Design review of the part built by this model. Coordinates are the model's own, in mm. A direction names the side the tool comes from. Give positions to 0.01 mm unless a question says otherwise; leave off trailing zeros. Order: outer loops, then holes, each group sorted by start corner. A loop starts at its lowest first (then second) coordinate and runs counter-clockwise, first axis right, second up. Notation, with made-up numbers: (83.25, -10) -> (139.25, -10) arc R30 cw to (139.25, 14) -> close; hole circle Ø7 at (29.25, 7.5). An arc over 180 degrees is marked (long way). Return JSON: item names as keys, results as strings.
```python
from build123d import *

# Parameters (mm, degrees)
SKETCH_1_W          = 16.3
SKETCH_1_H          = 31.2
SKETCH_1_R          = 3.05
SKETCH_1_R_2        = 1.05
SKETCH_1_R_3        = 2.55
EXTRUDE_1_DEPTH     = 2.5
SKETCH_2_R          = 1
CUT_EXTRUDE_1_DEPTH = 1
SKETCH_2_3_R        = 0.7
CUT_EXTRUDE_2_DEPTH = 21.5655051
SKETCH_3_R          = 1.5
SKETCH_3_R_2        = 2.5
EXTRUDE_2_DEPTH     = 9
CUT_EXTRUDE_START   = 9
SKETCH_3_3_R        = 0.3
CUT_EXTRUDE_3_DEPTH = 2
SKETCH_4_R          = 0.3
CUT_EXTRUDE_4_DEPTH = 2


with BuildPart() as part:
    # 草图1 → 凸台-拉伸1 (new body)
    with BuildSketch(Plane(origin=(0, 0, 0), x_dir=(1, 0, 0), z_dir=(0, 1, 0))):
        with Locations((3.15, 1.4)):
            Rectangle(SKETCH_1_W, SKETCH_1_H)
        with Locations(Location((0, 0, 0), (0, 0, 270))):
            Circle(SKETCH_1_R, mode=Mode.SUBTRACT)
        with Locations(Location((5.25646039, -8.152277238, 0), (0, 0, 270))):
            Circle(SKETCH_1_R_2, mode=Mode.SUBTRACT)
        with Locations(Location((6.4, -3.8, 0), (0, 0, 270))):
            Circle(SKETCH_1_R, mode=Mode.SUBTRACT)
        with Locations(Location((-0.337099263, 6.891760594, 0), (0, 0, 270))):
            Circle(SKETCH_1_R_3, mode=Mode.SUBTRACT)
        with Locations(Location((4.7, 11, 0), (0, 0, 270))):
            Circle(SKETCH_1_R_3, mode=Mode.SUBTRACT)
    extrude(amount=EXTRUDE_1_DEPTH)

    # 草图2 → 切除-拉伸1 (cut)
    with BuildSketch(Plane(origin=(0, 2.5, 0), x_dir=(1, 0, 0), z_dir=(0, 1, 0))):
        with Locations(Location((-3.5, 15.5, 0), (0, 0, 270))):
            Circle(SKETCH_2_R)
        with Locations(Location((-3.5, -12.7, 0), (0, 0, 270))):
            Circle(SKETCH_2_R)
        with Locations(Location((9.8, -12.7, 0), (0, 0, 270))):
            Circle(SKETCH_2_R)
        with Locations(Location((9.8, 15.5, 0), (0, 0, 270))):
            Circle(SKETCH_2_R)
        with Locations(Location((-3.5, -6.5, 0), (0, 0, 270))):
            Circle(SKETCH_2_R)
        with Locations(Location((9.8, 0, 0), (0, 0, 270))):
            Circle(SKETCH_2_R)
        with Locations(Location((9.8, 6.5, 0), (0, 0, 270))):
            Circle(SKETCH_2_R)
    extrude(amount=-CUT_EXTRUDE_1_DEPTH, mode=Mode.SUBTRACT)

    # 草图2<3> → 切除-拉伸2 (cut, through all)
    with BuildSketch(Plane(origin=(0, 2.5, 0), x_dir=(1, 0, 0), z_dir=(0, 1, 0))):
        with Locations(Location((9.8, 15.5, 0), (0, 0, 270))):
            Circle(SKETCH_2_3_R)
        with Locations(Location((9.8, -12.7, 0), (0, 0, 270))):
            Circle(SKETCH_2_3_R)
        with Locations(Location((-3.5, -12.7, 0), (0, 0, 270))):
            Circle(SKETCH_2_3_R)
        with Locations(Location((-3.5, 15.5, 0), (0, 0, 270))):
            Circle(SKETCH_2_3_R)
        with Locations(Location((-3.5, -6.5, 0), (0, 0, 270))):
            Circle(SKETCH_2_3_R)
        with Locations(Location((9.8, 0, 0), (0, 0, 270))):
            Circle(SKETCH_2_3_R)
        with Locations(Location((9.8, 6.5, 0), (0, 0, 270))):
            Circle(SKETCH_2_3_R)
    extrude(amount=-CUT_EXTRUDE_2_DEPTH, mode=Mode.SUBTRACT)

    # 草图3 → 凸台-拉伸2 (add)
    with BuildSketch(Plane(origin=(0, 2.5, 0), x_dir=(1, 0, 0), z_dir=(0, 1, 0))):
        with Locations(Location((-3.5, -9.6, 0), (0, 0, 180))):
            Circle(SKETCH_3_R)
        with Locations(Location((-3.5, 12, 0), (0, 0, 180))):
            Circle(SKETCH_3_R)
        with Locations(Location((6.3, 4, 0), (0, 0, 90))):
            Circle(SKETCH_3_R_2)
        with Locations((9.8, 11)):
            Circle(SKETCH_3_R)
    extrude(amount=EXTRUDE_2_DEPTH)

    # 草图3<3> → 切除-拉伸3 (cut)
    with BuildSketch(Plane(origin=(0, 2.5, 0), x_dir=(1, 0, 0), z_dir=(0, 1, 0)).offset(CUT_EXTRUDE_START)):
        with Locations(Location((-3.5, -9.6, 0), (0, 0, 270))):
            Circle(SKETCH_3_3_R)
        with Locations(Location((-3.5, 12, 0), (0, 0, 270))):
            Circle(SKETCH_3_3_R)
        with Locations(Location((6.3, 4, 0), (0, 0, 270))):
            Circle(SKETCH_3_3_R)
        with Locations(Location((9.8, 11, 0), (0, 0, 270))):
            Circle(SKETCH_3_3_R)
    extrude(amount=-CUT_EXTRUDE_3_DEPTH, mode=Mode.SUBTRACT)

    # 草图4 → 切除-拉伸4 (cut)
    with BuildSketch(Plane(origin=(0, 0, -17), x_dir=(-1, 0, 0), z_dir=(0, 0, -1))):
        with Locations((0.8, 1.187263162)):
            Circle(SKETCH_4_R)
        with Locations((-4.2, 1.187263162)):
            Circle(SKETCH_4_R)
    extrude(amount=-CUT_EXTRUDE_4_DEPTH, mode=Mode.SUBTRACT)


solid = part.part
```
Item 1: Add section B-B (z = 0). Give the boundary of the cut face in (x, y).
Result set:
{"outline": "(-5, 0) -> (-3.05, 0) -> (-3.05, 2.5) -> (-5, 2.5) -> close; (3.05, 0) -> (9.1, 0) -> (9.1, 1.5) -> (8.8, 1.5) -> (8.8, 2.5) -> (3.05, 2.5) -> close; (10.5, 0) -> (11.3, 0) -> (11.3, 2.5) -> (10.8, 2.5) -> (10.8, 1.5) -> (10.5, 1.5) -> close"}
Item 2: Machinability: for faces 4 (the face through (-3.2, 2.007, -14.546)), 5 (the face through (-4, 11.5, 10)), which of the approach directions +Z, -Z, +X, -X, +Y, -Y give a long, thin tool a straight path to every point of the face, cutting with its end or side? Answer none if there is none.
Result set:
{"face 4": "+Y", "face 5": "+Z, -Z, +X, -X, +Y"}
Item 3: Add section D-D (x = 0). Give the boundary of the cut face in (y, z).
Result set:
{"outline": "(0, -17) -> (2.5, -17) -> (2.5, -9.42) -> (0, -9.42) -> close; (0, -4.36) -> (2.5, -4.36) -> (2.5, -3.05) -> (0, -3.05) -> close; (0, 3.05) -> (2.5, 3.05) -> (2.5, 14.2) -> (0, 14.2) -> close"}
Item 4: Wall thickness on L1, parallel to X at y = 0.5, z = 0; L2, parallel to X at y = 0.6, z = 12.7; L3, parallel to X at y = 10.35, z = -4: over which ranges is each line inside the solid? List them lowest first. Write a range as [from, to].
Result set:
{"L1": "x = [-5, -3.05], [3.05, 9.1], [10.5, 11.3]", "L2": "x = [-5, -4.2], [-2.8, 9.1], [10.5, 11.3]", "L3": "x = [3.8, 6], [6.6, 8.8]"}
Item 5: For pin 1 (4 mm diameter, centred on x = -2, z = -0.5, fed in from +Y); pin 2 (0.7 mm diameter, centred on x = -3.5, z = -12, fed in from +Y); pin 3 (1.5 mm diameter, centred on x = 7.5, y = 9, fed in from -Z), all flat-tipped, find the tip position at first contact; note any pin that passes through.
Result set:
{"pin 1": "stops at y = 2.5", "pin 2": "stops at y = 11.5", "pin 3": "stops at z = -6.46"}
Item 6: Mouldability with a two-part tool opening along X and no side actions: class faces 1 (the face through (-5, 1, -1)), 2 (the face through (9, 11.5, -11)), 3 (the face through (9.424, 1.232, 3.403)) as released by +X, released by -X, zero draft, split by the parting line, or undercut.
Result set:
{"face 1": "released by -X", "face 2": "zero draft", "face 3": "undercut"}
Item 7: Add section C-C (y = 6.75). Give the boundary of the cut face in (x, z).
Result set:
{"outline": "circle Ø3 at (-3.5, -12); circle Ø3 at (-3.5, 9.6); circle Ø5 at (6.3, -4); circle Ø3 at (9.8, -11)"}
Item 8: Add section A-A (z = 3.8). Give the boundary of the cut face in (x, y), plus the area to 3 significant figures.
Result set:
{"outline": "(-5, 0) -> (3.35, 0) -> (3.35, 2.5) -> (-5, 2.5) -> close; (9.45, 0) -> (11.3, 0) -> (11.3, 2.5) -> (9.45, 2.5) -> close", "area": "25.5 mm^2"}
